Design review of the part shown in the three views and the two pictorial views. Dimensions are in mm from the part's minimum x, y and z. A direction names the side the tool comes from. Coordinates: 2 decimals unless noted, no trailing zeros. Loops run counter-clockwise (first coordinate to the right, second up) from the corner with the lowest first, then second, coordinate; pieces in that order, holes last. Notation, with made-up numbers: (15.5, 22) -> (52.5, 22) arc R18 cw to (52.5, 43) -> close; hole circle Ø7 at (-28, 0). An arc over 180 degrees is marked (long way). Answer in a Markdown table with one row per item.
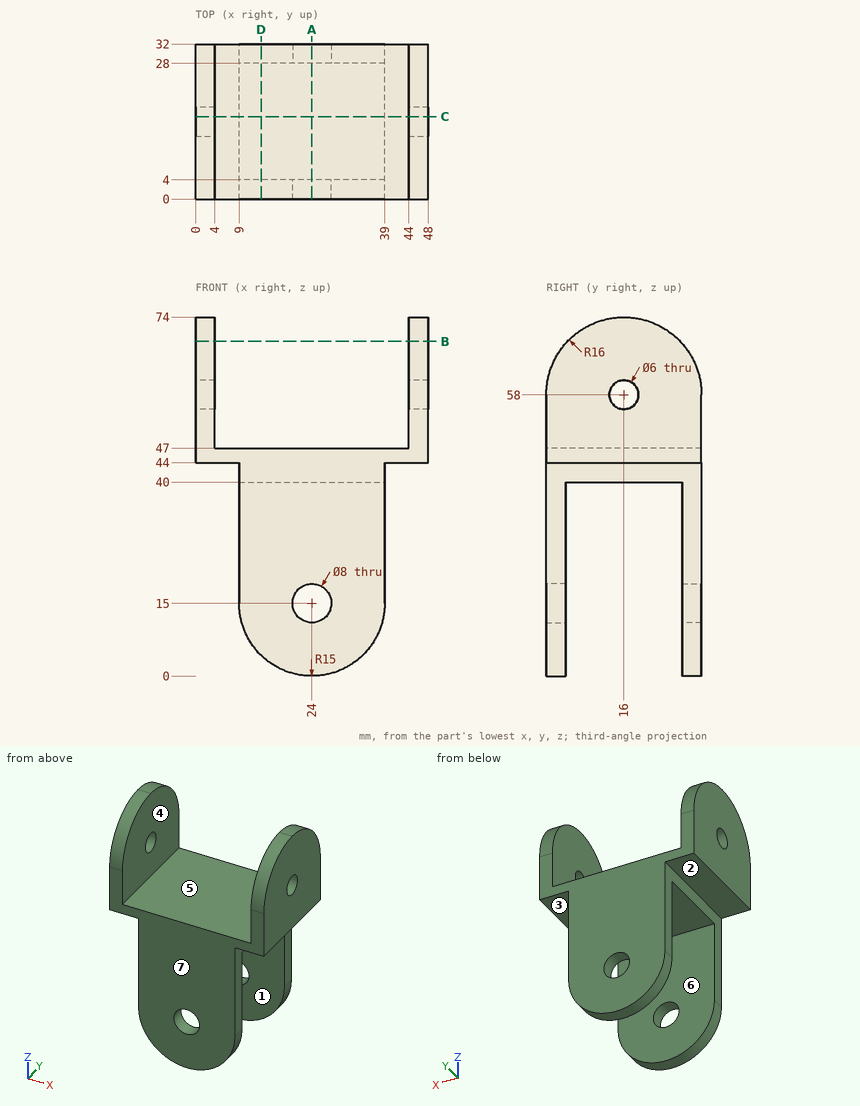
(1) To check wall thickness, follow probe 1 along Y at (x, z) = (26, 30.5); probe 2 along Z at (x, y) = (45.65, 16); probe 3 along X at (y, z) = (30, 15). State the ranges of each line that lie inside material, in increasing order.
Evaluation:
| item | result |
|---|---|
| probe 1 | y = 0 to 4, 28 to 32 |
| probe 2 | z = 44 to 55, 61 to 74 |
| probe 3 | x = 9 to 20, 28 to 39 |
(2) For pin 1 (8 mm diameter, centred on x = 30, y = 18, fed in from -Z); pin 2 (12 mm diameter, centred on x = 12.5, y = 13.5, fed in from +Z); pin 3 (10 mm diameter, centred on y = 10, z = 15.5, fed in from -X); pin 4 (2.5 mm diameter, centred on x = 4, y = 9.5, fed in from -Z), all flat-tipped, find the tip position at first contact; note any pin that passes through.
Evaluation:
| item | result |
|---|---|
| pin 1 | stops at z = 40 |
| pin 2 | stops at z = 47 |
| pin 3 | passes through |
| pin 4 | stops at z = 44 |
(3) Draft analysis for pull direction Y (two halves, no side actions). For the marked faces 5, 6 and 7, state which applies: pulls with the +Y half, pulls with the -Y half, needs draft (parallel to the pull), parting line crosses it, or undercut.
Evaluation:
| item | result |
|---|---|
| face 5 | needs draft |
| face 6 | undercut |
| face 7 | pulls with the -Y half |
(4) Take a section at A-A on x = 24. Give the boundary of the cut face in (y, z), and give its area (3 significant figures).
Evaluation:
| item | result |
|---|---|
| outline | (0, 0) -> (4, 0) -> (4, 11) -> (0, 11) -> close; (0, 19) -> (4, 19) -> (4, 40) -> (28, 40) -> (28, 19) -> (32, 19) -> (32, 47) -> (0, 47) -> close; (28, 0) -> (32, 0) -> (32, 11) -> (28, 11) -> close |
| area | 480 mm² |
(5) Take a section at C-C on y = 17. Give the boundary of the cut face in (x, z).
Evaluation:
| item | result |
|---|---|
| outline | (0, 44) -> (9, 44) -> (9, 40) -> (39, 40) -> (39, 44) -> (48, 44) -> (48, 55.17) -> (44, 55.17) -> (44, 47) -> (4, 47) -> (4, 55.17) -> (0, 55.17) -> close; (0, 60.83) -> (4, 60.83) -> (4, 73.97) -> (0, 73.97) -> close; (44, 60.83) -> (48, 60.83) -> (48, 73.97) -> (44, 73.97) -> close |
(6) Tool access review of the marked faces 1, 2, 3 and 4: name each direction out of +Z, -Z, +X, -X, +Y, -Y from which nothing blocks a thin tool from reaching the whole face with its end or side.
Evaluation:
| item | result |
|---|---|
| face 1 | -Z, +X, -X |
| face 2 | -Z, -X, +Y, -Y |
| face 3 | -Z, +X, +Y, -Y |
| face 4 | +Z, +Y, -Y |
(7) Take a section at B-B on z = 69. Give the boundary of the cut face in (x, y).
Evaluation:
| item | result |
|---|---|
| outline | (0, 4.38) -> (4, 4.38) -> (4, 27.62) -> (0, 27.62) -> close; (44, 4.38) -> (48, 4.38) -> (48, 27.62) -> (44, 27.62) -> close |
(8) Take a section at D-D on x = 13.5. Give the boundary of the cut face in (y, z).
Evaluation:
| item | result |
|---|---|
| outline | (0, 4.29) -> (4, 4.29) -> (4, 40) -> (28, 40) -> (28, 4.29) -> (32, 4.29) -> (32, 47) -> (0, 47) -> close |
